Here's how the part is built. I have some questions about the finished solid (model axes, mm). A direction names the side the tool comes from. Round coordinates to 2 decimals unless told otherwise and drop trailing zeros. Loops run counter-clockwise (first coordinate to the right, second up) from the corner with the lowest first, then second, coordinate; pieces in that order, holes last. Notation, with made-up numbers: M -33,58.25 L -23,58.25 A17 cw -23,70.25 Z; hole C 60.5,60.25 d6. An arc over 180 degrees is marked long. Use a Markdown table: item, result.
Autodesk Inventor part; units mm, degrees
ref_plane "YZ Plane" through (0, 0, 0) normal (1, 0, 0) x (0, 1, 0)
ref_plane "XZ Plane" through (0, 0, 0) normal (0, 1, 0) x (-1, 0, 0)
ref_plane "XY Plane" through (0, 0, 0) normal (0, 0, 1) x (1, 0, 0)
sketch "Sketch1" plane through (0, 0, 0) normal (0, 0, 1) x (1, 0, 0)
  line L0 (0, 0) -> (-6, 0)
  line L1 (-6, 0) -> (-30.5134, 20.5692)
  line L2 (-19.5134, 44) -> (-19.5134, 19.1716)
  line L3 (-19.5134, 19.1716) -> (-3.8162, 6)
  line L4 (0, 0) -> (0, 7.1987)
  circle A0 centre (-5.4048, 4.2) radius 0.889
  circle A1 centre (-22.8134, 18.1692) radius 0.889
  line L5 (-30.5134, 20.5692) -> (-25.4999, 20.5692)
  line L6 (-25.4999, 20.5692) -> (-25.4999, 26.5692)
  line L7 (-25.4999, 26.5692) -> (-29.4999, 26.5692)
  line L8 (-29.4999, 26.5692) -> (-29.4999, 41.5692)
  line L9 (-29.4999, 41.5692) -> (-25.4999, 41.5692)
  line L10 (-25.4999, 41.5692) -> (-25.4999, 50)
  line L11 (-25.4999, 50) -> (-15.8296, 50)
  line L12 (-15.8296, 50) -> (0, 36.7174)
  line L13 (-3, 31.4022) -> (-3, 6)
  line L14 (0, 7.1987) -> (0, 36.7174)
  line L15 (-18.0134, 44) -> (-3, 31.4022)
  line L16 (-19.5134, 44) -> (-18.0134, 44)
  line L17 (-3.8162, 6) -> (-3, 6)
  line L18 (0, 0) -> (6, 0)
  circle A2 centre (5.4048, 4.2) radius 0.889
  line L19 (19.5134, 19.1716) -> (3.8162, 6)
  line L20 (19.5134, 44) -> (19.5134, 19.1716)
  line L21 (6, 0) -> (30.5134, 20.5692)
  circle A3 centre (22.8134, 18.1692) radius 0.889
  line L22 (30.5134, 20.5692) -> (25.4999, 20.5692)
  line L23 (25.4999, 20.5692) -> (25.4999, 26.5692)
  line L24 (25.4999, 26.5692) -> (29.4999, 26.5692)
  line L25 (29.4999, 26.5692) -> (29.4999, 41.5692)
  line L26 (29.4999, 41.5692) -> (25.4999, 41.5692)
  line L27 (25.4999, 41.5692) -> (25.4999, 50)
  line L28 (25.4999, 50) -> (15.8296, 50)
  line L29 (15.8296, 50) -> (0, 36.7174)
  line L30 (3, 31.4022) -> (3, 6)
  line L31 (18.0134, 44) -> (3, 31.4022)
  line L32 (19.5134, 44) -> (18.0134, 44)
  line L33 (3.8162, 6) -> (3, 6)
  dimension "d0" = 6
  dimension "d2" = 40
  dimension "d5" = 1.778
  dimension "d6" = 32
  dimension "d8" = 3.3
  dimension "d9" = 2.4
  dimension "d10" = 4.2
  dimension "d11" = 6
  dimension "d13" = 5.0135
  dimension "d14" = 2.4
  dimension "d21" = 6
  dimension "d22" = 6
  dimension "d23" = 1.5
  dimension "d24" = 15
  dimension "d25" = 4
  dimension "d30" = 6
  dimension "d32" = 6
  dimension "d33" = 6
  dimension "d34" = 5.9865
  dimension "d35" = 50
extrude "Extrusion1" add sketch "Sketch1" along normal mid plane 8
properties part number "Leg_part2"
1. Imagine slicing it at C-C, the plane y = 4.2. Write out the boundary of the cut face in (x, z), then the cut area to 3 significant figures.
Answer sheet:
| item | result |
|---|---|
| outline | M -11.01,-4 L -6.29,-4 L -6.29,4 L -11.01,4 Z; M -4.52,-4 L 4.52,-4 L 4.52,4 L -4.52,4 Z; M 6.29,-4 L 11.01,-4 L 11.01,4 L 6.29,4 Z |
| area | 148 mm2 |
2. We'd pull the mould along X, two halves only. Please class faces 4 (the face through (21, 50, 0)), 5 (the face through (-25.5, 24, 0)), 6 (the face through (-6.06, 3.6, -0.06)): +X half, -X half, draft (parallel to the pull), parting line (faces both ways), or undercut.
Answer sheet:
| item | result |
|---|---|
| face 4 | draft |
| face 5 | -X half |
| face 6 | undercut |
3. Imagine slicing it at D-D, the plane z = 1.75. State how many separate pieces and enclosed holes the cut face has, then the cut area to 3 significant figures.
Answer sheet:
| item | result |
|---|---|
| separate pieces | 1 |
| enclosed holes | 6 |
| area | 1,290 mm2 |
4. Imagine slicing it at B-B, the plane x = -23. Write out the boundary of the cut face in (y, z), then the cut area to 3 significant figures.
Answer sheet:
| item | result |
|---|---|
| outline | M 14.26,-4 L 17.3,-4 L 17.3,4 L 14.26,4 Z; M 19.04,-4 L 50,-4 L 50,4 L 19.04,4 Z |
| area | 272 mm2 |
5. Which directions (+Z, -Z, +X, -X, +Y, -Y) give clear straight access to the entire face, cutting with the end or side of a thin tool? Please do faces 1 (the face through (27, 26.569, 0)), 2 (the face through (-10.61, 37.79, -0.06)), 3 (the face through (29.5, 34, 0)).
Answer sheet:
| item | result |
|---|---|
| face 1 | +Z, -Z, +X |
| face 2 | +Z, -Z |
| face 3 | +Z, -Z, +X, +Y |
6. For pin 1 Ø2.5 at (x, y) = (-5.4, 4.2) entering from -Z; pin 2 Ø2.5 at (y, z) = (37, -0.5) entering from -X; pin 3 Ø1.6 at (x, z) = (-19, -1) entering from -Y; pin 4 Ø4 at (y, z) = (45, 0) entering from +X, each with a flat end and sliding along its axis, tell me the tip position at first contact or that it passes through.
Answer sheet:
| item | result |
|---|---|
| pin 1 | z = -4 |
| pin 2 | x = -29.5 |
| pin 3 | y = 10.24 |
| pin 4 | x = 25.5 |
7. Imagine slicing it at A-A, the plane y = 16. Write out the boundary of the cut face in (x, z), then the cut area to 3 significant figures.
Answer sheet:
| item | result |
|---|---|
| outline | M -25.07,-4 L -15.73,-4 L -15.73,4 L -25.07,4 Z; M -3,-4 L 3,-4 L 3,4 L -3,4 Z; M 15.73,-4 L 25.07,-4 L 25.07,4 L 15.73,4 Z |
| area | 197 mm2 |
8. I need wall thicknesses on probe 1 along X at (y, z) = (29.5, 1); probe 2 along Y at (x, z) = (-5, 1.5); probe 3 along X at (y, z) = (43, 2.75). Which ranges of each line are inside material? Lowest first, please. Write a range as from..to.
Answer sheet:
| item | result |
|---|---|
| probe 1 | -29.5..-19.51, -3..3, 19.51..29.5 |
| probe 2 | 0..3.41, 4.99..6.99, 33.08..40.91 |
| probe 3 | -25.5..-19.51, -16.82..-7.49, 7.49..16.82, 19.51..25.5 |
